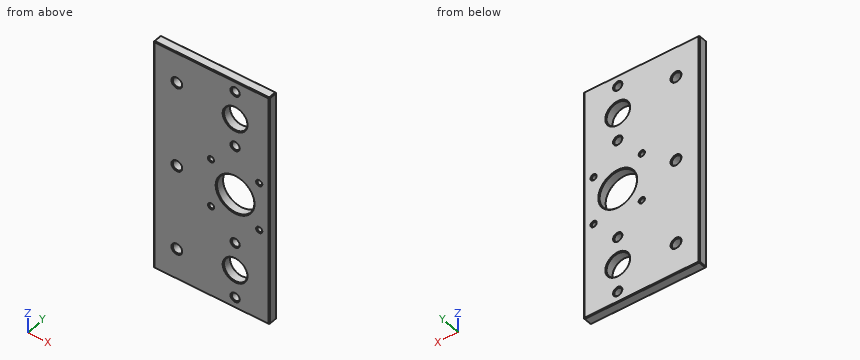
from build123d import *

# Parameters (mm, degrees)
CROQUIS1_W              = 74.5
CROQUIS1_H              = 150
CROQUIS1_R              = 1.5
CROQUIS1_R_2            = 3
CROQUIS1_R_3            = 12
CROQUIS1_R_4            = 7.5
CROQUIS1_R_5            = 2.5
SALIENTE_EXTRUIR1_DEPTH = 6
CHAFL_N1_SIZE           = 0.5


with BuildPart() as part:
    # Croquis1 → Saliente-Extruir1 (new body)
    with BuildSketch(Plane(origin=(0, 0, 0), x_dir=(1, 0, 0), z_dir=(0, 1, 0))):
        with Locations((-2.478313692, -1.041413592)):
            Rectangle(CROQUIS1_W, CROQUIS1_H)
        with Locations(Location((-2.728313692, 14.458586408, 0), (0, 0, 270))):
            Circle(CROQUIS1_R, mode=Mode.SUBTRACT)
        with Locations(Location((28.271686308, 14.458586408, 0), (0, 0, 270))):
            Circle(CROQUIS1_R, mode=Mode.SUBTRACT)
        with Locations(Location((-2.728313692, -16.541413592, 0), (0, 0, 270))):
            Circle(CROQUIS1_R, mode=Mode.SUBTRACT)
        with Locations(Location((28.271686308, -16.541413592, 0), (0, 0, 270))):
            Circle(CROQUIS1_R, mode=Mode.SUBTRACT)
        with Locations(Location((-24.728313692, 53.958586408, 0), (0, 0, 270))):
            Circle(CROQUIS1_R_2, mode=Mode.SUBTRACT)
        with Locations(Location((-24.728313692, -56.041413592, 0), (0, 0, 270))):
            Circle(CROQUIS1_R_2, mode=Mode.SUBTRACT)
        with Locations(Location((12.771686308, -1.041413592, 0), (0, 0, 270))):
            Circle(CROQUIS1_R_3, mode=Mode.SUBTRACT)
        with Locations(Location((-24.728313692, -1.041413592, 0), (0, 0, 270))):
            Circle(CROQUIS1_R_2, mode=Mode.SUBTRACT)
        with Locations(Location((12.771686308, -51.041413592, 0), (0, 0, 270))):
            Circle(CROQUIS1_R_4, mode=Mode.SUBTRACT)
        with Locations(Location((12.771686308, 48.958586408, 0), (0, 0, 270))):
            Circle(CROQUIS1_R_4, mode=Mode.SUBTRACT)
        with Locations(Location((12.771686308, 66.958586408, 0), (0, 0, 270))):
            Circle(CROQUIS1_R_5, mode=Mode.SUBTRACT)
        with Locations(Location((12.771686308, 30.958586408, 0), (0, 0, 270))):
            Circle(CROQUIS1_R_5, mode=Mode.SUBTRACT)
        with Locations(Location((12.771686308, -33.041413592, 0), (0, 0, 270))):
            Circle(CROQUIS1_R_5, mode=Mode.SUBTRACT)
        with Locations(Location((12.771686308, -69.041413592, 0), (0, 0, 270))):
            Circle(CROQUIS1_R_5, mode=Mode.SUBTRACT)
    extrude(amount=SALIENTE_EXTRUIR1_DEPTH)

    # Chafl_n1
    chafl_n1_edges = [part.edges().sort_by_distance(p)[0] for p in [
        (34.771686308, 6, 1.041413592),
        (-2.728313692, 0, -15.958586408),
        (-2.728313692, 6, -15.958586408),
        (-2.478313692, 6, -73.958586408),
        (28.271686308, 0, -15.958586408),
        (28.271686308, 6, -15.958586408),
        (-2.728313692, 0, 15.041413592),
        (-2.728313692, 6, 15.041413592),
        (28.271686308, 0, 15.041413592),
        (28.271686308, 6, 15.041413592),
        (-24.728313692, 0, -56.958586408),
        (-24.728313692, 6, -56.958586408),
        (-24.728313692, 0, 53.041413592),
        (-24.728313692, 6, 53.041413592),
        (12.771686308, 0, -10.958586408),
        (12.771686308, 6, -10.958586408),
        (-24.728313692, 0, -1.958586408),
        (-24.728313692, 6, -1.958586408),
        (-39.728313692, 6, 1.041413592),
        (12.771686308, 0, 43.541413592),
        (12.771686308, 6, 43.541413592),
        (-2.478313692, 0, -73.958586408),
        (12.771686308, 0, -56.458586408),
        (12.771686308, 6, -56.458586408),
        (34.771686308, 0, 1.041413592),
        (12.771686308, 0, -69.458586408),
        (12.771686308, 6, -69.458586408),
        (-2.478313692, 0, 76.041413592),
        (12.771686308, 0, -33.458586408),
        (12.771686308, 6, -33.458586408),
        (-39.728313692, 0, 1.041413592),
        (12.771686308, 0, 30.541413592),
        (12.771686308, 6, 30.541413592),
        (12.771686308, 0, 66.541413592),
        (12.771686308, 6, 66.541413592),
        (-2.478313692, 6, 76.041413592),
        (-39.728313692, 3, -73.958586408),
        (34.771686308, 3, -73.958586408),
        (34.771686308, 3, 76.041413592),
        (-39.728313692, 3, 76.041413592),
    ]]
    chamfer(chafl_n1_edges, length=CHAFL_N1_SIZE)


solid = part.part
The listing builds one solid part. Answer for the finished solid, in the listing's coordinates (mm). Give positions to 0.01 mm unless a question says otherwise; leave off trailing zeros.
Item 1: Find the intervals of material crossed by line 1 along Z through (x, y) = (-2.5, 1); line 2 along X through (y, z) = (1.75, -67); line 3 along Z through (x, y) = (7.5, 4), in increasing order.
Derived:
line 1: z = -73.96 to -15.94, -12.98 to 15.06, 18.02 to 76.04
line 2: x = -39.73 to 10.27, 15.27 to 34.77
line 3: z = -73.96 to -54.29, -43.62 to -9.74, 11.82 to 45.71, 56.38 to 76.04
Item 2: Each of these flat-tipped pins is pushed along its axis until it touches: pin 1 Ø1.5 at (x, z) = (6, 12.5) entering from -Y; pin 2 Ø3.5 at (x, z) = (28.27, 16.54) entering from +Y. Where does it stop, or does it pass through?
Derived:
pin 1: stops at y = 0
pin 2: stops at y = 5.75
Item 3: A cutting plane is placed at A-A (y = 4). Give the number of separate pieces and of enclosed holes in the cut face, then the cut area to 3 significant figures.
Derived:
separate pieces: 1
enclosed holes: 14
area: 10,200 mm2
